from build123d import *

# Parameters (mm, degrees)
BOSS_EXTRUDE1_DEPTH = 11.5
FILLET1_R           = 5
SKETCH2_R           = 16
BOSS_EXTRUDE2_DEPTH = 508
FILLET2_R           = 1
SKETCH4_R           = 17.5
BOSS_EXTRUDE3_DEPTH = 29
CHAMFER1_SIZE       = 3.5
SKETCH5_R           = 14
BOSS_EXTRUDE4_DEPTH = 508
SKETCH6_R           = 14.5
BOSS_EXTRUDE5_DEPTH = 34
CHAMFER2_SIZE       = 3.5
SKETCH7_R           = 13
BOSS_EXTRUDE6_DEPTH = 8
SKETCH8_R           = 3.175
BOSS_EXTRUDE7_DEPTH = 12
SKETCH9_R           = 11.5
BOSS_EXTRUDE8_DEPTH = 12
FILLET3_R           = 9


with BuildPart() as part:
    # Sketch1 → Boss-Extrude1 (new body, symmetric)
    with BuildSketch(Plane.XY):
        with BuildLine():
            Line((-33.008488745, -30.177022886), (-48.008488745, -30.177022886))
            Line((-48.008488745, -30.177022886), (-56.008488745, -42.865600426))
            Line((-56.008488745, -42.865600426), (-56.008488745, -49.440306382))
            Line((-56.008488745, -49.440306382), (-46.767158149, -40.808664634))
            ThreePointArc((-46.767158149, -40.808664634), (-39.008488745, -42.177022886), (-46.767158149, -43.545381137))
            Line((-46.767158149, -43.545381137), (-56.008488745, -52.177022886))
            Line((-56.008488745, -52.177022886), (-53.008488745, -52.177022886))
            Line((-53.008488745, -52.177022886), (-53.008488745, -54.177022886))
            Line((-53.008488745, -54.177022886), (-56.008488745, -54.177022886))
            Line((-56.008488745, -54.177022886), (-56.008488745, -56.177022886))
            Line((-56.008488745, -56.177022886), (-54.008488745, -56.177022886))
            Line((-54.008488745, -56.177022886), (-54.008488745, -58.177022886))
            Line((-54.008488745, -58.177022886), (-35.008488745, -58.177022886))
            Line((-35.008488745, -58.177022886), (-35.008488745, -56.177022886))
            Line((-35.008488745, -56.177022886), (-33.008488745, -56.177022886))
            Line((-33.008488745, -56.177022886), (-33.008488745, -30.177022886))
        make_face()
    extrude(amount=BOSS_EXTRUDE1_DEPTH, both=True)

    # Fillet1
    fillet1_edges = [part.edges().sort_by_distance(p)[0] for p in [
        (-48.008488745, -30.177022886, 0),
        (-33.008488745, -30.177022886, 0),
        (-56.008488745, -42.865600426, 0),
    ]]
    fillet(fillet1_edges, radius=FILLET1_R)

    # Sketch2 → Boss-Extrude2 (add)
    with BuildSketch(Plane(origin=(0, -58.177022886, 0), x_dir=(-1, 0, 0), z_dir=(0, -1, 0))):
        with Locations((44.508488745, -0.100800937)):
            Circle(SKETCH2_R)
    extrude(amount=BOSS_EXTRUDE2_DEPTH)

    # Fillet2
    fillet2_edges = [part.edges().sort_by_distance(p)[0] for p in [
        (-28.508488745, -58.177022886, 0.100800937),
    ]]
    fillet(fillet2_edges, radius=FILLET2_R)

    # Sketch4 → Boss-Extrude3 (add)
    with BuildSketch(Plane(origin=(0, -566.177022886, 0), x_dir=(-1, 0, 0), z_dir=(0, -1, 0))):
        with Locations((44.508488745, -0.100800937)):
            Circle(SKETCH4_R)
    extrude(amount=BOSS_EXTRUDE3_DEPTH)

    # Chamfer1
    chamfer1_edges = [part.edges().sort_by_distance(p)[0] for p in [
        (-27.008488745, -595.177022886, 0.100800937),
    ]]
    chamfer(chamfer1_edges, length=CHAMFER1_SIZE)

    # Sketch5 → Boss-Extrude4 (add)
    with BuildSketch(Plane(origin=(0, -595.177022886, 0), x_dir=(-1, 0, 0), z_dir=(0, -1, 0))):
        with Locations((44.508488745, -0.100800937)):
            Circle(SKETCH5_R)
    extrude(amount=BOSS_EXTRUDE4_DEPTH)

    # Sketch6 → Boss-Extrude5 (add)
    with BuildSketch(Plane.XZ.offset(1103.177022886)):
        with Locations((-44.508488745, 0.100800937)):
            Circle(SKETCH6_R)
    extrude(amount=BOSS_EXTRUDE5_DEPTH)

    # Chamfer2
    chamfer2_edges = [part.edges().sort_by_distance(p)[0] for p in [
        (-59.008488745, -1137.177022886, 0.100800937),
    ]]
    chamfer(chamfer2_edges, length=CHAMFER2_SIZE)

    # Sketch7 → Boss-Extrude6 (add)
    with BuildSketch(Plane.XZ.offset(1137.177022886)):
        with Locations((-44.508488745, 0.100800937)):
            Circle(SKETCH7_R)
    extrude(amount=BOSS_EXTRUDE6_DEPTH)

    # Sketch8 → Boss-Extrude7 (add)
    with BuildSketch(Plane.XZ.offset(1145.177022886)):
        with Locations((-44.508488745, 0.100800937)):
            Circle(SKETCH8_R)
    extrude(amount=BOSS_EXTRUDE7_DEPTH)

    # Sketch9 → Boss-Extrude8 (add)
    with BuildSketch(Plane(origin=(0, -1157.177022886, 0), x_dir=(-1, 0, 0), z_dir=(0, -1, 0))):
        with Locations((44.508488745, -0.100800937)):
            Circle(SKETCH9_R)
    extrude(amount=BOSS_EXTRUDE8_DEPTH)

    # Fillet3
    fillet3_edges = [part.edges().sort_by_distance(p)[0] for p in [
        (-33.008488745, -1169.177022886, 0.100800937),
    ]]
    fillet(fillet3_edges, radius=FILLET3_R)


solid = part.part
Geometry check sheet. Reference: the model listing, model coordinates, mm. A direction names the side the tool comes from. Round coordinates to 2 decimals unless told otherwise and drop trailing zeros. Order: outer loops, then holes, each group sorted by start corner. A loop starts at its lowest first (then second) coordinate and runs counter-clockwise, first axis right, second up. Notation, with made-up numbers: M 69.25,24 L 98.25,24 A19 ccw 98.25,35 Z; hole C 49.5,-5.5 d4. An arc over 180 degrees is marked long. Answer in a Markdown table with one row per item. Add a question column.
Item 1: Set-up check for faces 1 (the face through (-33.008, -46, 0)), 2 (the face through (-42, -1145.177, -3)), 3 (the face through (-45, -47, 11.5)): record each of +Z, -Z, +X, -X, +Y, -Y from which the full face is reachable in a straight line by a thin tool's end or side.
Item 2: Material ranges on L1, parallel to Y at x = -40.5, z = 1; L2, parallel to Y at x = -48, z = -7; L3, parallel to Z at x = -47, y = -245.5, recorded low to high. Write a range as [from, to].
Item 3: Depth check by flat-ended pin: pin 1 Ø10 at (x, y) = (-55, -490.5) entering from +Z; pin 2 Ø10 at (y, z) = (-598, -0.5) entering from -X; pin 3 Ø9 at (x, y) = (-43.01, -42.18) entering from +Z; pin 4 Ø8 at (x, z) = (-44.5, -5) entering from -Y. Enter the tip coordinate at first touch or a pass-through.
Item 4: Sectioned sample at A-A, the plane y = -1045.5. Enter the section's corners in (x, z), plus the area to 3 significant figures.
Filled in:
| question | item | result |
|---|---|---|
| 1 | face 1 | +Z, -Z, +X, +Y |
| 1 | face 2 | none |
| 1 | face 3 | +Z, +X, -X, +Y |
| 2 | L1 | y = [-1169.03, -1157.18], [-1145.18, -45.29], [-39.06, -30.18] |
| 2 | L2 | y = [-1167.37, -1157.18], [-1145.18, -44.7], [-41.96, -31] |
| 2 | L3 | z = [-15.7, 15.91] |
| 3 | pin 1 | stops at z = 15.13 |
| 3 | pin 2 | stops at x = -60.68 |
| 3 | pin 3 | stops at z = 11.5 |
| 3 | pin 4 | stops at y = -1169.18 |
| 4 | outline | C -44.51,0.1 d28 |
| 4 | area | 616 mm² |
